from build123d import *

# Parameters (mm, degrees)
BOSS_EXTRUDE1_DEPTH = 55
CUT_EXTRUDE4_DEPTH  = 3
CUT_EXTRUDE5_DEPTH  = 3


with BuildPart() as part:
    # Sketch3 → Boss-Extrude1 (new body)
    with BuildSketch(Plane.XY):
        Polygon((-76.265076845, 1.199033895), (-77.169023428, -1.284538931), (77.169023428, -1.284538931), (76.265076845, 1.199033895), (76.233955557, 1.284538931), (76.075119575, 1.284538931), (-76.233955557, 1.284538931), align=None)
    extrude(amount=-BOSS_EXTRUDE1_DEPTH)

    # Sketch4 → Cut-Extrude4 (cut)
    with BuildSketch(Plane(origin=(0, 1.284538931, 0), x_dir=(1, 0, 0), z_dir=(0, 1, 0))):
        Polygon((-14.9, 0), (-14.9, 37), (14.9, 37), (14.9, 0.115445968), (14.9, -2.514676192), (-14.9, -2.514676192), align=None)
    extrude(amount=-CUT_EXTRUDE4_DEPTH, mode=Mode.SUBTRACT)

    # Sketch5 → Cut-Extrude5 (cut)
    with BuildSketch(Plane(origin=(0, 1.284538931, 0), x_dir=(1, 0, 0), z_dir=(0, 1, 0))):
        with BuildLine():
            Line((-60.900466668, 23.5), (-30.233488889, 23.5))
            ThreePointArc((-30.233488889, 23.5), (-25.233488889, 18.5), (-30.233488889, 13.5))
            Line((-30.233488889, 13.5), (-60.900466668, 13.5))
            ThreePointArc((-60.900466668, 13.5), (-65.900466668, 18.5), (-60.900466668, 23.5))
        make_face()
        with BuildLine():
            Line((60.900466668, 13.5), (30.233488889, 13.5))
            ThreePointArc((30.233488889, 13.5), (25.233488889, 18.5), (30.233488889, 23.5))
            Line((30.233488889, 23.5), (60.900466668, 23.5))
            ThreePointArc((60.900466668, 23.5), (65.900466668, 18.5), (60.900466668, 13.5))
        make_face()
    extrude(amount=-CUT_EXTRUDE5_DEPTH, mode=Mode.SUBTRACT)


solid = part.part
Verification items for the finished model (mm, model axes). A direction names the side the tool comes from. Round coordinates to 2 decimals unless told otherwise and drop trailing zeros. Order: outer loops, then holes, each group sorted by start corner. A loop starts at its lowest first (then second) coordinate and runs counter-clockwise, first axis right, second up.
1. Section check C-C on z = -18.5. Record the cut outline in (x, y), then the cut area to 3 significant figures.
Final values:
outline: (-77.17, -1.28) - (-65.9, -1.28) - (-65.9, 1.28) - (-76.23, 1.28) - close; (-25.23, -1.28) - (-14.9, -1.28) - (-14.9, 1.28) - (-25.23, 1.28) - close; (14.9, -1.28) - (25.23, -1.28) - (25.23, 1.28) - (14.9, 1.28) - close; (65.9, -1.28) - (77.17, -1.28) - (76.23, 1.28) - (65.9, 1.28) - close
area: 109 mm2
2. Section check B-B on z = -33.5. Record the cut outline in (x, y), then the cut area to 3 significant figures.
Final values:
outline: (-77.17, -1.28) - (-14.9, -1.28) - (-14.9, 1.28) - (-76.23, 1.28) - close; (14.9, -1.28) - (77.17, -1.28) - (76.23, 1.28) - (14.9, 1.28) - close
area: 318 mm2
3. Thickness scan on L1, parallel to Z at x = -39.5, y = 0.95; L2, parallel to X at y = 0.75, z = -22; L3, parallel to X at y = 1.2, z = -34.5. Record the ranges inside material, lowest first.
Final values:
L1: z = -55 to -23.5, -13.5 to 0
L2: x = -76.43 to -64.47, -26.66 to -14.9, 14.9 to 26.66, 64.47 to 76.43
L3: x = -76.26 to -14.9, 14.9 to 76.26
4. Go/stop test with flat-tipped pins: P1, Ø4, axis at x = -5, z = -33.5, coming from the +Y side; P2, Ø1.3, axis at x = -0.5, y = 0.5, coming from the +Z side. Record where each tip stops, or that it passes through.
Final values:
P1: passes through
P2: stops at z = -37
5. Section check D-D on y = 0.1. Record the cut outline in (x, z), then the cut area to 3 significant figures.
Final values:
outline: (-76.67, -55) - (76.67, -55) - (76.67, 0) - (14.9, 0) - (14.9, -37) - (-14.9, -37) - (-14.9, 0) - (-76.67, 0) - close; hole (-60.9, -23.5) - (-30.23, -23.5) arc R5 ccw to (-30.23, -13.5) - (-60.9, -13.5) arc R5 ccw to start; hole (30.23, -23.5) - (60.9, -23.5) arc R5 ccw to (60.9, -13.5) - (30.23, -13.5) arc R5 ccw to start
area: 6,560 mm2
6. Release check for a two-part mould opening along X. For faces 4 (the flat face through (1, 1.285, -39)), 5 (the cylindrical face through (25.235, 0.018, -18.39)) record: +X half, -X half, draft (parallel to the pull), parting line (faces both ways), or undercut.
Final values:
face 4: draft
face 5: undercut
7. Section check A-A on x = -58.5. Record the cut outline in (y, z).
Final values:
outline: (-1.28, -55) - (1.28, -55) - (1.28, -23.5) - (-1.28, -23.5) - close; (-1.28, -13.5) - (1.28, -13.5) - (1.28, 0) - (-1.28, 0) - close
8. Access from +Z, -Z, +X, -X, +Y, -Y to the whole of each face (thin tool, end or side, straight path). Record for faces 1 (the flat face through (14.9, 0, -18)), 2 (the flat face through (-1, -1.285, -39)), 3 (the flat face through (46, 0, -13.5)).
Final values:
face 1: +Z, +Y, -Y
face 2: +Z, -Z, +X, -X, -Y
face 3: +Y, -Y
